Work out the finished part from the listing and answer in its coordinate system (mm). A direction names the side the tool comes from. Round coordinates to 2 decimals unless told otherwise and drop trailing zeros. Write each loop counter-clockwise with the first axis right and the second up, starting at its lowest first coordinate (ties: lowest second). Pieces come first, ordered by that corner, then holes. Notation, with made-up numbers: (10, -10.75) -> (17, -10.75) arc R25 ccw to (17, 19.25) -> close; hole circle Ø11 at (1.25, -15.75). An arc over 180 degrees is marked (long way). Answer as a JSON object with one key per item and string values. Group by question number.
Autodesk Fusion 360 part; units mm, degrees
sketch "Sketch1" plane through (0, 0, 0) normal (0, 0, 1) x (1, 0, 0)
  circle A0 centre (0, 0) radius 2.5
  dimension "d1" = 5
extrude "Extrude1" add sketch "Sketch1" along normal blind 6
sketch "Sketch2" plane through (0, 0, 6) normal (0, 0, 1) x (-1, 0, 0)
  circle A0 centre (0, 0) radius 2.5
  circle A1 centre (0, 0) radius 1.5
  dimension "d4" = 3
extrude "Extrude2" cut sketch "Sketch2" against normal blind 5 contours A1
sketch "Sketch3" plane through (0, 0, 1) normal (0, 0, 1) x (-1, 0, 0)
  circle A0 centre (0, 0) radius 1.5
  line L0 (1.2625, -0.8099) -> (-1.2492, -0.8303)
  arc A1 (0.0066, -1.5) -> (-1.2492, -0.8303) centre (0, 0) ccw
extrude "Extrude3" add sketch "Sketch3" along normal blind 5 contours A0 L0 A1 picked at (0.6944, -1.19)
1) A cutting plane is placed at B-B on x = 0. Determine the outline of the cut face in (y, z).
2) A cutting plane is placed at C-C on z = 3.3. Determine the outline of the cut face in (x, y).
3) A tool of negligible diameter and unlimited length cuts with its end or side. For faces 1 (the face through (0, -1.5, 3.5)), 2 (the face through (0, 0, 0)), from which of +Z, -Z, +X, -X, +Y, -Y can it reach the whole face along a straight path? Write none if from no direction.
4) A cutting plane is placed at D-D on y = 1.1. Determine the outline of the cut face in (x, z) (3 decimals), plus the area to 3 significant figures.
5) A cutting plane is placed at A-A on y = 0. Determine the outline of the cut face in (x, z), plus the area to 3 significant figures.
6) Straight lines are drawn through the part: L1, parallel to Y at x = 0.5, z = 4; L2, parallel to Y at x = 0, z = 4.2; L3, parallel to Z at x = -1.3, y = -0.35. For each, find the intervals that lie inside material, in ascending order.
7) Each of these flat-tipped pins is pushed along its axis until it touches: P1, Ø1.5, axis at y = 1.5, z = 0.5, coming from the -X side; P2, Ø1.5, axis at x = -0.5, y = 0.5, coming from the -Z side; P3, Ø1.2, axis at x = 0, y = 0, coming from the +Z side; P4, Ø1.5, axis at y = 1, z = 4, coming from the +X side. Where does it stop, or does it pass through?
8) For a pull along X with two mould halves and no side action, classify faces 3 (the face through (0, 1, 6)), 4 (the face through (-0.54, 2.44, 2.96)), 5 (the face through (0, 0, 1)) as released by +X, released by -X, zero draft, split by the parting line, or undercut.
Established:
{
 "1": {"outline": "(-2.5, 0) -> (2.5, 0) -> (2.5, 6) -> (0.82, 6) -> (0.82, 1) -> (-1.5, 1) -> (-1.5, 6) -> (-2.5, 6) -> close"},
 "2": {"outline": "circle Ø5 at (0, 0); hole (-1.26, 0.81) arc R1.5 ccw (long way) to (1.25, 0.83) -> close"},
 "3": {"face 1": "+Z", "face 2": "-Z, +X, -X, +Y, -Y"},
 "4": {"outline": "(-2.245, 0) -> (2.245, 0) -> (2.245, 6) -> (-2.245, 6) -> close", "area": "26.9 mm²"},
 "5": {"outline": "(-2.5, 0) -> (2.5, 0) -> (2.5, 6) -> (1.5, 6) -> (1.5, 1) -> (-1.5, 1) -> (-1.5, 6) -> (-2.5, 6) -> close", "area": "15.0 mm²"},
 "6": {"L1": "y = -2.45 to -1.41, 0.82 to 2.45", "L2": "y = -2.5 to -1.5, 0.82 to 2.5", "L3": "z = 0 to 1"},
 "7": {"P1": "stops at x = -2.38", "P2": "stops at z = 0", "P3": "stops at z = 1", "P4": "stops at x = 2.49"},
 "8": {"face 3": "zero draft", "face 4": "split by the parting line", "face 5": "undercut"}
}
